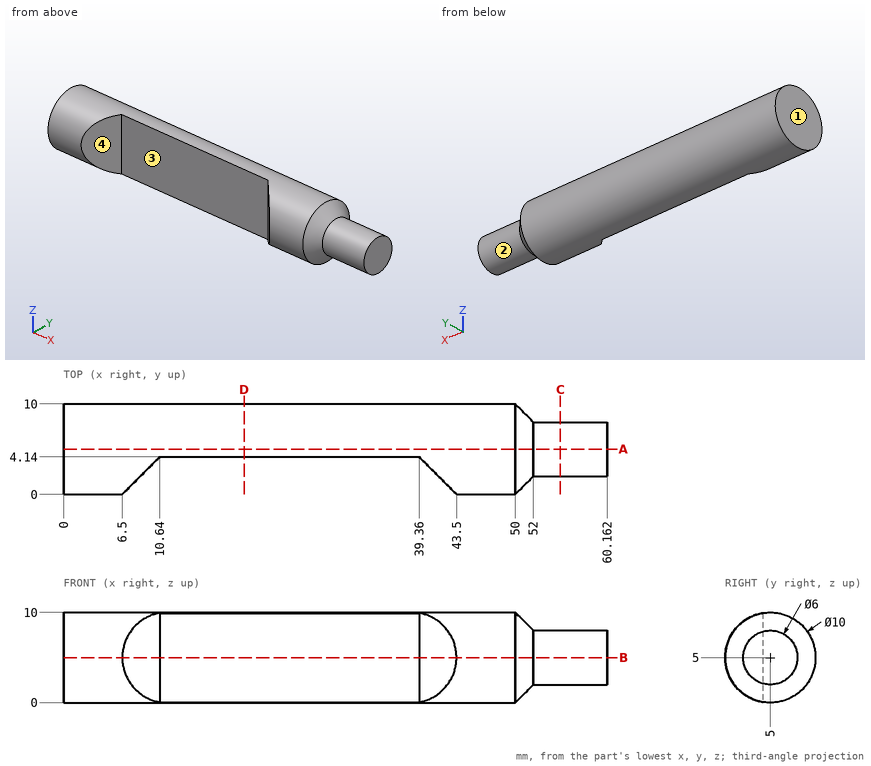
Print and shaded views of the part. All mm, measured from the part's lowest x, y and z. Coordinates: 2 decimals unless noted, no trailing zeros. Loops run counter-clockwise (first coordinate to the right, second up) from the corner with the lowest first, then second, coordinate; pieces in that order, holes last. Notation, with made-up numbers: (49, 51.5) - (104, 51.5) arc R20 cw to (104, 62.5) - close; hole circle Ø10 at (81.25, 8.5). An arc over 180 degrees is marked (long way). Use one line per item in the form item = value. Start each with the question number.
1) Two-plate mould, pull along X, no slides. Class the marked faces 1, 2, 3 and 4: +X half, -X half, draft (parallel to the pull), parting line (faces both ways), or undercut.
2) Band-saw the part on B-B (z = 5). Give the cut face in (x, y), and give its area (3 significant figures).
3) Band-saw the part on A-A (y = 5). Give the cut face in (x, z), and give its area (3 significant figures).
4) Band-saw the part on C-C (x = 55). Give the cut face in (y, z).
5) Band-saw the part on D-D (x = 20). Give the cut face in (y, z).
6) Drill centre lines: L1, parallel to Y at x = 3.5, z = 9; L2, parallel to X at y = 4, z = 5.75; L3, parallel to Z at x = 57.5, y = 4.75. Where is each one in solid material? Low to high. Write a range as from..to.
7) Flat gauge pins, fed straight in: pin 1 (1 mm diameter, centred on y = 8.5, z = 3.5, fed in from +X); pin 2 (1.5 mm diameter, centred on x = 36, y = 9, fed in from -Z); pin 3 (1 mm diameter, centred on x = 47, z = 3, fed in from +Y). Where does each tip first touch, or does it go through?
Check values:
q1.face_1 = -X half
q1.face_2 = draft
q1.face_3 = undercut
q1.face_4 = undercut
q2.outline = (0, 0) - (6.5, 0) - (10.64, 4.14) - (39.36, 4.14) - (43.5, 0) - (50, 0) - (52, 2) - (60.16, 2) - (60.16, 8) - (52, 8) - (50, 10) - (0, 10) - close
q2.area = 429 mm2
q3.outline = (0, 0) - (50, 0) - (52, 2) - (60.16, 2) - (60.16, 8) - (52, 8) - (50, 10) - (0, 10) - close
q3.area = 565 mm2
q4.outline = circle Ø6 at (5, 5)
q5.outline = (4.14, 0.07) arc R5 ccw (long way) to (4.14, 9.93) - close
q6.L1 = 2..8
q6.L2 = 0..10.5, 39.5..60.16
q6.L3 = 2.01..7.99
q7.pin_1 = 51.69
q7.pin_2 = 1.2
q7.pin_3 = 9.77
